Answer from the drawing. Dimensions are ordinates in mm from the lowest x, y and z of the part. A direction names the side the tool comes from. Coordinates: 2 decimals unless noted, no trailing zeros. Write each loop counter-clockwise with the first axis right and the second up, starting at its lowest first coordinate (ties: lowest second). Pieces come first, ordered by that corner, then holes. Notation, with made-up numbers: (74, 20) - (105, 20) arc R19 ccw to (105, 53) - close; hole circle Ø3 at (-8, -27). An arc over 180 degrees is marked (long way). Use one line per item in the form item = value. Start each with the question number.
Item 1: For the marked faces 1, 2 and 3, determine the directions among +Z, -Z, +X, -X, +Y, -Y from which every point of the face is accessible in a straight line to the end or side of a thin tool.
Item 2: Given pin 1 (4 mm diameter, centred on y = 3.5, z = 26, fed in from +X); pin 2 (2.5 mm diameter, centred on y = 5, z = 26, fed in from -X); pin 3 (2.5 mm diameter, centred on x = 41.5, y = 5.5, fed in from +Z), each flat-ended and moving along its own axis, determine where each tip first touches the part or whether it passes through.
Item 3: A cutting plane is placed at C-C (z = 16). Write down the section's boundary in (x, y), then the cut area to 3 significant figures.
Item 4: Determine the mould class of the marked faces 4, 5 and 6 for opening direction X: released by +X, released by -X, zero draft, split by the parting line, or undercut.
Item 5: A cutting plane is placed at B-B (y = 4.25). Give the number of separate pieces and of enclosed holes in the cut face, then the cut area to 3 significant figures.
Item 6: A cutting plane is placed at A-A (x = 5). Write down the section's boundary in (y, z).
Item 7: Consider probe 1 along X at (y, z) = (4.25, 49); probe 2 along Y at (x, z) = (5, 49); probe 3 along X at (y, z) = (2, 20). Determine where each line is inside the solid, lowest interval first.
Item 8: A cutting plane is placed at D-D (x = 16.35). Write down the section's boundary in (y, z).
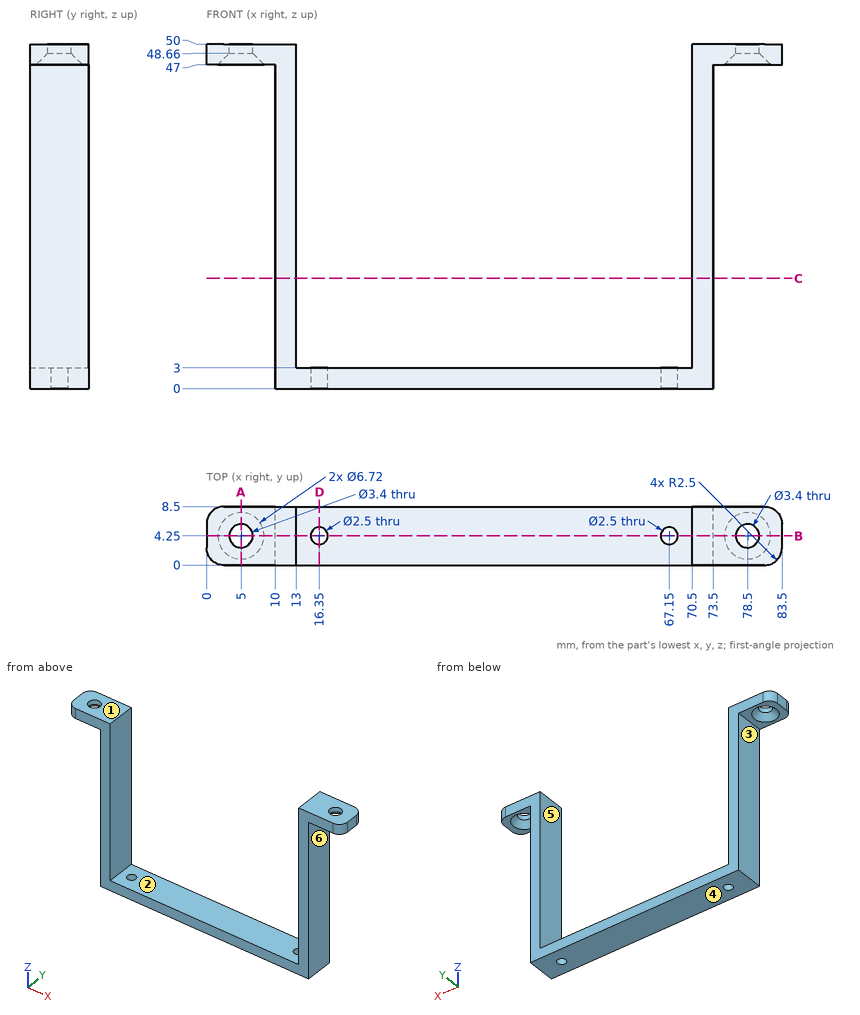
Answer:
q1.face_1 = +Z, +X, -X, +Y, -Y
q1.face_2 = +Z, +Y, -Y
q1.face_3 = -Z, -X, +Y, -Y
q2.pin_1 = 73.5
q2.pin_2 = 10
q2.pin_3 = 3
q3.outline = (10, 0) - (13, 0) - (13, 8.5) - (10, 8.5) - close; (70.5, 0) - (73.5, 0) - (73.5, 8.5) - (70.5, 8.5) - close
q3.area = 51.0 mm²
q4.face_4 = zero draft
q4.face_5 = undercut
q4.face_6 = released by +X
q5.separate_pieces = 5
q5.enclosed_holes = 0
q5.area = 492 mm²
q6.outline = (0, 47) - (0.89, 47) - (2.55, 48.66) - (2.55, 50) - (0, 50) - close; (5.95, 48.66) - (7.61, 47) - (8.5, 47) - (8.5, 50) - (5.95, 50) - close
q7.probe_1 = 0 to 3.3, 6.7 to 13, 70.5 to 76.8, 80.2 to 83.5
q7.probe_2 = 0 to 2.55, 5.95 to 8.5
q7.probe_3 = 10 to 13, 70.5 to 73.5
q8.outline = (0, 0) - (3, 0) - (3, 3) - (0, 3) - close; (5.5, 0) - (8.5, 0) - (8.5, 3) - (5.5, 3) - close
